Answer from the drawing. Dimensions are ordinates in mm from the lowest x, y and z of the part. A direction names the side the tool comes from. Give positions to 0.01 mm unless a question says otherwise; leave off trailing zeros. Loops run counter-clockwise (first coordinate to the right, second up) from the corner with the lowest first, then second, coordinate; pieces in that order, holes last. Notation, with made-up numbers: (30, -3) - (65, -3) arc R33 ccw to (65, 28) - close; hole circle Ø6 at (30, 28.25). An arc over 180 degrees is marked (long way). Answer as CSV lines item,"result". Start each with the question number.
1) A cutting plane is placed at B-B (x = 14.89). Determine the outline of the cut face in (y, z), and give its area (3 significant figures).
2) A cutting plane is placed at D-D (y = 26). Determine the outline of the cut face in (x, z).
3) Flat-ended cylindrical pins translate along their axes: pin 1 (8 mm diameter, centred on y = 3.5, z = 6.5, fed in from +X); pin 2 (6 mm diameter, centred on x = 24.5, y = 23, fed in from -Z); pin 3 (0.7 mm diameter, centred on y = 7, z = 13.5, fed in from +X); pin 4 (3 mm diameter, centred on y = 5.5, z = 18.5, fed in from -X). Find the tip coordinate at first contact, or state that the pin passes through.
4) For a pull along X with two mould halves and no side action, classify the marked faces 1, 2 and 3 as pulls with the +X half, pulls with the -X half, needs draft (parallel to the pull), parting line crosses it, or undercut.
5) For the marked faces 4 and 5, determine the directions among +Z, -Z, +X, -X, +Y, -Y from which every point of the face is accessible in a straight line to the end or side of a thin tool.
6) A cutting plane is placed at C-C (y = 14.89). Determine the outline of the cut face in (x, z).
7) Find the intervals of material crossed by line 1 along X through (y, z) = (14.89, 24); line 2 along Y through (x, z) = (15.5, 8) (1 decimal); line 3 along X through (y, z) = (20.25, 18.5) (1 decimal), in increasing order.
8) A cutting plane is placed at A-A (z = 12). Determine the outline of the cut face in (x, y) (1 decimal).
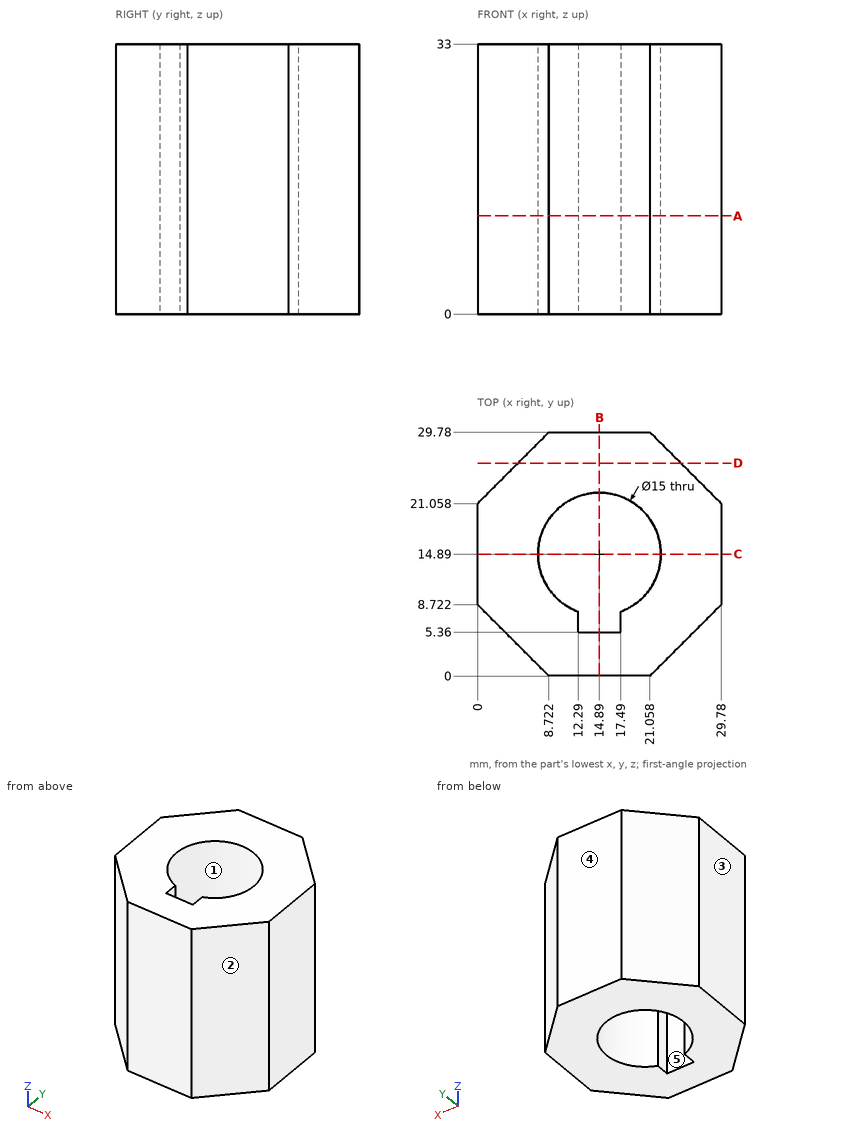
Ans:
1,outline,"(0, 0) - (5.36, 0) - (5.36, 33) - (0, 33) - close; (22.39, 0) - (29.78, 0) - (29.78, 33) - (22.39, 33) - close"
1,area,"421 mm2"
2,outline,"(4.94, 0) - (24.84, 0) - (24.84, 33) - (4.94, 33) - close"
3,pin 1,"x = 28.56"
3,pin 2,"z = 0"
3,pin 3,"x = 28.41"
3,pin 4,"x = 1.72"
4,face 1,"undercut"
4,face 2,"pulls with the +X half"
4,face 3,"pulls with the -X half"
5,face 4,"+Z, -Z, +X, -X, +Y"
5,face 5,"+Z, -Z"
6,outline,"(0, 0) - (7.39, 0) - (7.39, 33) - (0, 33) - close; (22.39, 0) - (29.78, 0) - (29.78, 33) - (22.39, 33) - close"
7,line 1,"0 to 7.39, 22.39 to 29.78"
7,line 2,"0 to 5.4, 22.4 to 29.8"
7,line 3,"0 to 9.6, 20.1 to 29.8"
8,outline,"(0, 8.7) - (8.7, 0) - (21.1, 0) - (29.8, 8.7) - (29.8, 21.1) - (21.1, 29.8) - (8.7, 29.8) - (0, 21.1) - close; hole (12.3, 5.4) - (17.5, 5.4) - (17.5, 7.9) arc R7.5 ccw (long way) to (12.3, 7.9) - close"
